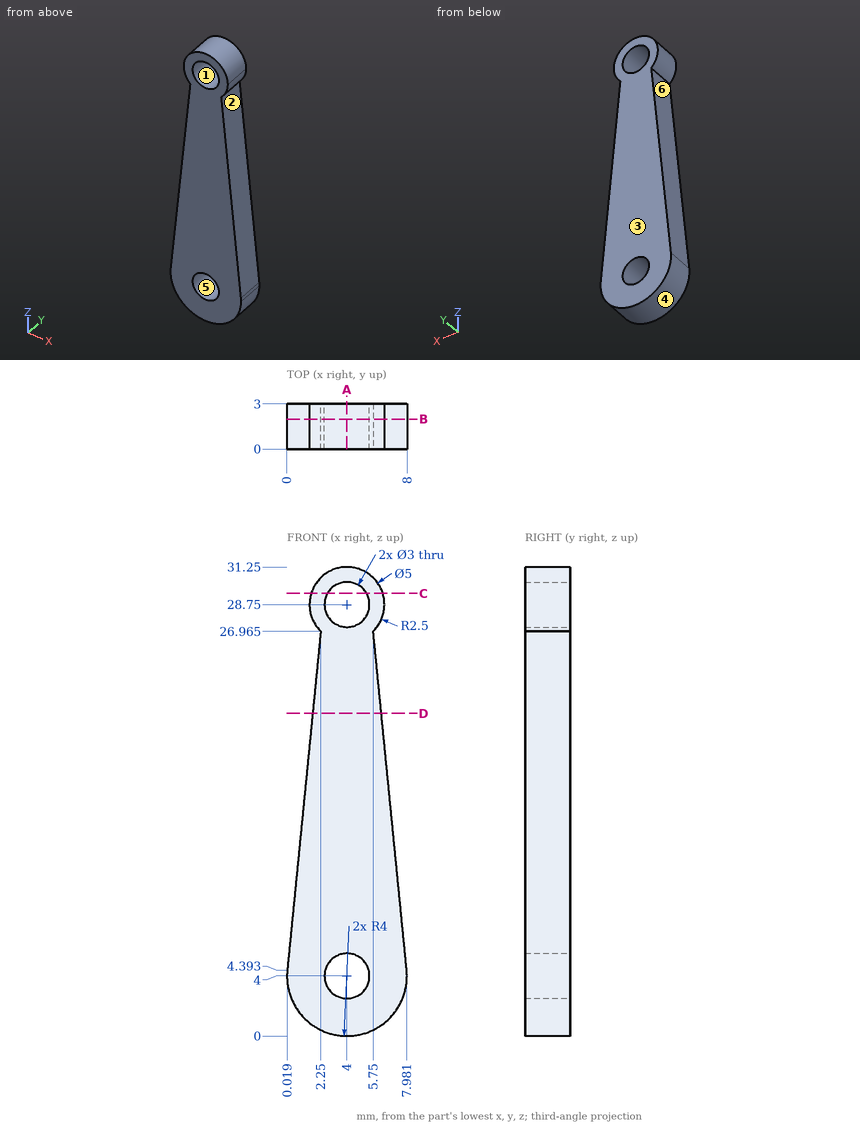
Source: three-view drawing plus pictorial views. Frame: mm from the lowest corner of the part. A direction names the side the tool comes from. Give positions to 0.01 mm unless a question says otherwise; leave off trailing zeros. Loops run counter-clockwise (first coordinate to the right, second up) from the corner with the lowest first, then second, coordinate; pieces in that order, holes last. Notation, with made-up numbers: (83.5, 79.25) -> (110.5, 79.25) arc R33 cw to (110.5, 114.25) -> close; hole circle Ø8 at (68.25, 75). An arc over 180 degrees is marked (long way). Use a Markdown table: item, result. Add a question column.
(1) First-contact query: pin 1 Ø1 at (x, y) = (6.5, 1) entering from +Z; pin 2 Ø1 at (y, z) = (2, 16) entering from -X; pin 3 Ø2.5 at (x, z) = (4, 28.75) entering from +Y (1 decimal); pin 4 Ø1.5 at (x, y) = (6, 1) entering from -Z. Flat tips, straight axial feed; report the tip coordinate or a pass-through.
(2) Pull-direction query (X, two-part tool) for the marked faces 3, 4, 5 and 6; classes: +X half, -X half, draft (parallel to the pull), parting line (faces both ways), or undercut.
(3) Section query B-B (y = 2). Count the separate pieces of the cut face and the enclosed holes in it, then the cut area to 3 significant figures.
(4) Ray query, line 1 (Z direction, x = 4, y = 1.8); line 2 (X direction, y = 2.3, z = 28.75); line 3 (Z direction, x = 3, y = 0.85) (1 decimal). Return the intervals inside material, ascending.
(5) Section query D-D (z = 21.5). Output: boundary loops of the cut face in (x, y).
(6) Section query A-A (x = 4). Output: boundary loops of the cut face in (y, z).
(7) Access query for the marked faces 1 and 2. Directions: +Z, -Z, +X, -X, +Y, -Y. A direction counts if a zero-diameter tool reaches every point of the face in a straight line with its end or side. Return the directions, or none.
(8) Section query C-C (z = 29.5). Output: boundary loops of the cut face in (x, y) (1 decimal).
Checked values:
| question | item | result |
|---|---|---|
| 1 | pin 1 | z = 30.25 |
| 1 | pin 2 | x = 1.12 |
| 1 | pin 3 | through |
| 1 | pin 4 | z = 0.2 |
| 2 | face 3 | draft |
| 2 | face 4 | parting line |
| 2 | face 5 | undercut |
| 2 | face 6 | -X half |
| 3 | separate pieces | 1 |
| 3 | enclosed holes | 2 |
| 3 | area | 161 mm^2 |
| 4 | line 1 | 0 to 2.5, 5.5 to 27.25, 30.25 to 31.25 |
| 4 | line 2 | 1.5 to 2.5, 5.5 to 6.5 |
| 4 | line 3 | 0.1 to 2.9, 5.1 to 27.6, 29.9 to 31 |
| 5 | outline | (1.71, 0) -> (6.29, 0) -> (6.29, 3) -> (1.71, 3) -> close |
| 6 | outline | (0, 0) -> (3, 0) -> (3, 2.5) -> (0, 2.5) -> close; (0, 5.5) -> (3, 5.5) -> (3, 27.25) -> (0, 27.25) -> close; (0, 30.25) -> (3, 30.25) -> (3, 31.25) -> (0, 31.25) -> close |
| 7 | face 1 | +Y, -Y |
| 7 | face 2 | +X, +Y, -Y |
| 8 | outline | (1.6, 0) -> (2.7, 0) -> (2.7, 3) -> (1.6, 3) -> close; (5.3, 0) -> (6.4, 0) -> (6.4, 3) -> (5.3, 3) -> close |
